from build123d import *

# Parameters (mm, degrees)
RESSALTO_EXTRUS_O1_DEPTH = 4
FURO_COM_FOLGA_DE_M41_D  = 4.5


with BuildPart() as part:
    # Esboço1 → Ressalto-extrusão1 (new body)
    with BuildSketch(Plane(origin=(0, 0, 0), x_dir=(1, 0, 0), z_dir=(0, 1, 0))):
        Polygon((30, -78.75), (55, -78.75), (55, 78.75), (-55, 78.75), (-55, -78.75), (-30, -78.75), (-30, -48.75), (30, -48.75), align=None)
    extrude(amount=RESSALTO_EXTRUS_O1_DEPTH)

    # Furo com folga de M41 (through all)
    with Locations(Plane(origin=(0, 4, 0), x_dir=(1, 0, 0), z_dir=(0, 1, 0))):
        with Locations((-45, 63.75), (45, 63.75), (45, -63.75), (-45, -63.75)):
            Hole(FURO_COM_FOLGA_DE_M41_D / 2)


solid = part.part
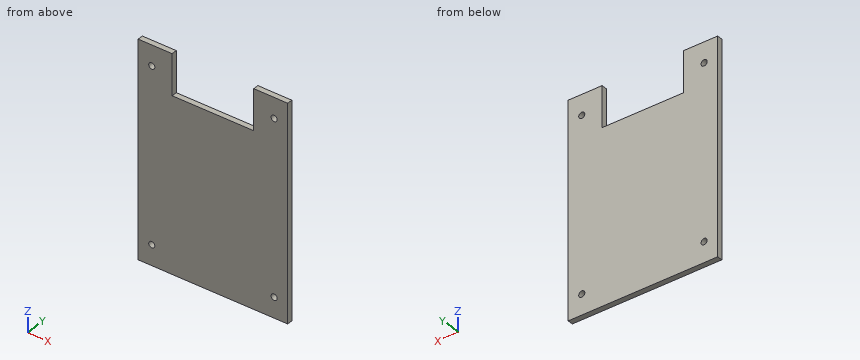
For this review, take the finished solid that the model builds, in its own axes (mm). Coordinates: 2 decimals unless noted, no trailing zeros. Order: outer loops, then holes, each group sorted by start corner. A loop starts at its lowest first (then second) coordinate and runs counter-clockwise, first axis right, second up. Notation, with made-up numbers: (70, 31) - (120, 31) arc R19 cw to (120, 36) - close; hole circle Ø7 at (34, 57.25). An arc over 180 degrees is marked (long way). Answer as CSV lines item,"result". Start each with the question number.
1) Insertion check: P1, Ø1, axis at x = 18, y = 3, coming from the +Z side; P2, Ø2.5, axis at x = -45, z = -63.75, coming from the +Y side. Each pin has a flat end and moves straight along its axis. Give the tip position at first contact, or say it passes through.
2) To check wall thickness, follow line 1 along Z through (x, y) = (-45, 1.1); line 2 along X through (y, z) = (2, 64); line 3 along X through (y, z) = (1.35, 71.5). State the ranges of each line that lie inside material, in increasing order. Write a range as [from, to].
3) Add section A-A (x = 45). State the section outline as (y, z) points.
4) Add section C-C (z = -63.75). State the section outline as (x, y) points.
5) Add section B-B (z = 68.5). State the section outline as (x, y) points, then the cut area to 3 significant figures.
6) Add section D-D (y = 3.35). State the section outline as (x, z) points.
Result:
1,P1,"z = 48.75"
1,P2,"through"
2,line 1,"[-78.75, -66], [-61.5, 61.5], [66, 78.75]"
2,line 2,"[-55, -47.24], [-42.76, -30], [30, 42.76], [47.24, 55]"
2,line 3,"[-55, -30], [30, 55]"
3,outline,"(0, -78.75) - (4, -78.75) - (4, -66) - (0, -66) - close; (0, -61.5) - (4, -61.5) - (4, 61.5) - (0, 61.5) - close; (0, 66) - (4, 66) - (4, 78.75) - (0, 78.75) - close"
4,outline,"(-55, 0) - (-47.25, 0) - (-47.25, 4) - (-55, 4) - close; (-42.75, 0) - (42.75, 0) - (42.75, 4) - (-42.75, 4) - close; (47.25, 0) - (55, 0) - (55, 4) - (47.25, 4) - close"
5,outline,"(-55, 0) - (-30, 0) - (-30, 4) - (-55, 4) - close; (30, 0) - (55, 0) - (55, 4) - (30, 4) - close"
5,area,"200 mm^2"
6,outline,"(-55, -78.75) - (55, -78.75) - (55, 78.75) - (30, 78.75) - (30, 48.75) - (-30, 48.75) - (-30, 78.75) - (-55, 78.75) - close; hole circle Ø4.5 at (-45, -63.75); hole circle Ø4.5 at (-45, 63.75); hole circle Ø4.5 at (45, -63.75); hole circle Ø4.5 at (45, 63.75)"
